Autodesk Inventor part; units mm, degrees
ref_plane "YZ Plane" through (0, 0, 0) normal (1, 0, 0) x (0, 1, 0)
ref_plane "XZ Plane" through (0, 0, 0) normal (0, 1, 0) x (-1, 0, 0)
ref_plane "XY Plane" through (0, 0, 0) normal (0, 0, 1) x (1, 0, 0)
sketch "Sketch1" plane through (0, 0, 0) normal (0, 0, 1) x (1, 0, 0)
  line L0 (0, 0) -> (25.4, 0)
  line L1 (25.4, 0) -> (25.4, 25.4)
  line L2 (0, 25.4) -> (0, 0)
  line L3 (3.175, 3.175) -> (22.225, 3.175)
  line L4 (22.225, 3.175) -> (22.225, 25.4)
  line L5 (3.175, 25.4) -> (3.175, 3.175)
  line L6 (25.4, 25.4) -> (22.225, 25.4)
  line L7 (3.175, 25.4) -> (0, 25.4)
  dimension "d0" = 25.4
  dimension "d1" = 25.4
  dimension "d2" = 3.175
  dimension "d3" = 3.175
  dimension "d4" = 3.175
extrude "Extrusion1" add sketch "Sketch1" along normal blind 25.4
sketch "Sketch2" plane through (25.4, 0, 0) normal (1, 0, 0) x (0, 0, -1)
  line L0 (-25.4, 25.4) -> (-25.4, 0)
  line L1 (0, 0) -> (-25.4, 0)
  line L2 (0, 0) -> (0, 25.4)
  line L3 (0, 25.4) -> (-25.4, 25.4)
  arc A0 (-6.7505, 21.2696) -> (-18.6495, 21.2696) centre (-12.7, 19.05) ccw
  circle A1 centre (-12.7, 19.05) radius 3.175
  line L4 (-25.4, 3.175) -> (-18.6495, 21.2696)
  line L5 (0, 3.175) -> (-6.7505, 21.2696)
  dimension "d7" = 19.05
  dimension "d8" = 12.7
  dimension "d9" = 6.35
  dimension "d10" = 3.175
  dimension "d11" = 3.175
extrude "Extrusion2" cut sketch "Sketch2" against normal blind 25.4 contours L3 A0 L4 L0 | L3 L2 L5 A0 | A1
equation "\"d1\" = d0"
equation "\"d3\" = d2"
equation "\"d4\" = d2"
equation "\"d11\" = d10"
properties part number "manipulator actuator braket"
Input: part model. Units: mm. Frame: model coordinates. A direction names the side the tool comes from. Round coordinates to 2 decimals unless told otherwise and drop trailing zeros. Loops run counter-clockwise (first coordinate to the right, second up) from the corner with the lowest first, then second, coordinate; pieces in that order, holes last. Notation, with made-up numbers: M 7,33.5 L 32,33.5 A16 ccw 32,51.5 Z; hole C -4.5,50 d10. An arc over 180 degrees is marked long. Answer in a Markdown table with one row per item. Add a question column.
1. Section C-C (y = 8.5). Output: boundary loops of the cut face in (x, z) (3 decimals), and give its area (3 significant figures).
2. Mould query, pull axis X, two halves, no side actions, for faces 1 (the face through (22.225, 12, 13)), 2 (the face through (1.61, 12.1, 22.07)), 3 (the face through (0, 10, 13)). Classes: released by +X, released by -X, zero draft, split by the parting line, or undercut.
3. Contact query for flat-ended pins moving along their axis: pin 1 (2 mm diameter, centred on x = 3.5, y = 8.5, fed in from +Z); pin 2 (5 mm diameter, centred on y = 19.05, z = 12.7, fed in from -X); pin 3 (2 mm diameter, centred on y = 7, z = 6, fed in from -X); pin 4 (12 mm diameter, centred on x = 21.5, y = 15, fed in from +Z). Output: stop coordinate, or through.
4. Section A-A (z = 12.7). Output: boundary loops of the cut face in (x, y) (3 decimals), and give its area (3 significant figures).
5. Section D-D (y = 19.05). Output: boundary loops of the cut face in (x, z) (3 decimals), and give its area (3 significant figures).
6. Ray query, probe 1 along Y at (x, z) = (0.75, 12.7) (3 decimals); probe 2 along X at (y, z) = (4.25, 24.25) (3 decimals); probe 3 along Y at (x, z) = (22, 16.25) (3 decimals). Return the intervals inside material, ascending.
7. Set-up query: faces 4 (the face through (1.6, 25.4, 12.6)), 5 (the face through (3.175, 12, 13)). Return all of +Z, -Z, +X, -X, +Y, -Y with unobstructed straight access to the full face (end or side cutting, diameter ignored); none if empty.
Values follow:
| question | item | result |
|---|---|---|
| 1 | outline | M 0,1.987 L 3.175,1.987 L 3.175,23.413 L 0,23.413 Z; M 22.225,1.987 L 25.4,1.987 L 25.4,23.413 L 22.225,23.413 Z |
| 1 | area | 136 mm^2 |
| 2 | face 1 | undercut |
| 2 | face 2 | zero draft |
| 2 | face 3 | released by -X |
| 3 | pin 1 | z = 23.77 |
| 3 | pin 2 | through |
| 3 | pin 3 | x = 0 |
| 3 | pin 4 | z = 23.21 |
| 4 | outline | M 0,0 L 25.4,0 L 25.4,15.875 L 22.225,15.875 L 22.225,3.175 L 3.175,3.175 L 3.175,15.875 L 0,15.875 Z; M 0,22.225 L 3.175,22.225 L 3.175,25.4 L 0,25.4 Z; M 22.225,22.225 L 25.4,22.225 L 25.4,25.4 L 22.225,25.4 Z |
| 4 | area | 181 mm^2 |
| 5 | outline | M 0,5.922 L 3.175,5.922 L 3.175,9.525 L 0,9.525 Z; M 0,15.875 L 3.175,15.875 L 3.175,19.478 L 0,19.478 Z; M 22.225,5.922 L 25.4,5.922 L 25.4,9.525 L 22.225,9.525 Z; M 22.225,15.875 L 25.4,15.875 L 25.4,19.478 L 22.225,19.478 Z |
| 5 | area | 45.8 mm^2 |
| 6 | probe 1 | 0 to 15.875, 22.225 to 25.4 |
| 6 | probe 2 | 0 to 3.175, 22.225 to 25.4 |
| 6 | probe 3 | 0 to 3.175 |
| 7 | face 4 | +X, -X, +Y |
| 7 | face 5 | +Z, -Z, +Y |
